Verification items for the finished model (mm, model axes). A direction names the side the tool comes from. Round coordinates to 2 decimals unless told otherwise and drop trailing zeros. Order: outer loops, then holes, each group sorted by start corner. A loop starts at its lowest first (then second) coordinate and runs counter-clockwise, first axis right, second up. Notation, with made-up numbers: (28.5, 59) -> (34.5, 59) arc R28 cw to (34.5, 77) -> close; hole circle Ø8 at (0.25, 37.5). An arc over 180 degrees is marked (long way). Put each result on its own line as item: value.
from build123d import *

# Parameters (mm, degrees)
SALIENTE_EXTRUIR1_DEPTH      = 2
SALIENTE_EXTRUIR3_DEPTH      = 2.5
SALIENTE_EXTRUIR3_DEPTH_BACK = 2
CROQUIS4_R                   = 1.5
SALIENTE_EXTRUIR4_DEPTH      = 2
CORTAR_EXTRUIR1_DEPTH        = 2


with BuildPart() as part:
    # Croquis1 → Saliente-Extruir1 (new body)
    with BuildSketch(Plane(origin=(0, 0, 0), x_dir=(1, 0, 0), z_dir=(0, 1, 0))):
        Polygon((-0.5, 44.6), (9.5, 54.6), (44.6, 54.6), (54.6, 44.6), (54.6, 9.5), (44.6, -0.5), (9.5, -0.5), (-0.5, 9.5), align=None)
    extrude(amount=SALIENTE_EXTRUIR1_DEPTH)

    # Croquis2 → Saliente-Extruir3 (add, two sides: drawn at the far end of the back side and taken through both)
    with BuildSketch(Plane(origin=(0, 2, 0), x_dir=(1, 0, 0), z_dir=(0, 1, 0)).offset(-SALIENTE_EXTRUIR3_DEPTH_BACK)):
        Polygon((7.5, 56.6), (-2.5, 46.6), (-2.5, 7.5), (7.5, -2.5), (46.6, -2.5), (56.6, 7.5), (56.6, 46.6), (46.6, 56.6), align=None)
        Polygon((44.6, -0.5), (9.5, -0.5), (-0.5, 9.5), (-0.5, 44.6), (9.5, 54.6), (44.6, 54.6), (54.6, 44.6), (54.6, 9.5), align=None, mode=Mode.SUBTRACT)
    extrude(amount=SALIENTE_EXTRUIR3_DEPTH + SALIENTE_EXTRUIR3_DEPTH_BACK)

    # Croquis4 → Saliente-Extruir4 (add)
    # profile 1 of 2: a face of its own
    with BuildSketch(Plane.XZ):
        with BuildLine():
            Line((13.025, 2.5), (21.525, 2.5))
            Line((21.525, 2.5), (21.525, 19.5))
            ThreePointArc((21.525, 19.5), (17.275, 23.75), (13.025, 19.5))
            Line((13.025, 19.5), (13.025, 2.5))
        make_face()
        with Locations(Location((17.275, 19.5, 0), (0, 0, 270))):
            Circle(CROQUIS4_R, mode=Mode.SUBTRACT)
    # profile 2 of 2: a face of its own
    with BuildSketch(Plane.XZ):
        with BuildLine():
            Line((32.575, 19.5), (32.575, 2.5))
            Line((32.575, 2.5), (41.075, 2.5))
            Line((41.075, 2.5), (41.075, 19.5))
            ThreePointArc((41.075, 19.5), (36.825, 23.75), (32.575, 19.5))
        make_face()
        with Locations(Location((36.825, 19.5, 0), (0, 0, 270))):
            Circle(CROQUIS4_R, mode=Mode.SUBTRACT)
    extrude(amount=-SALIENTE_EXTRUIR4_DEPTH)

    # Croquis6 → Cortar-Extruir1 (cut)
    with BuildSketch(Plane(origin=(0, 2, 0), x_dir=(1, 0, 0), z_dir=(0, 1, 0))):
        Polygon((4.5, 30.05), (24.05, 30.05), (24.05, 49.6), (9.5, 49.6), (4.5, 44.6), align=None)
        Polygon((30.05, 30.05), (30.05, 49.6), (44.6, 49.6), (49.6, 44.6), (49.6, 30.05), align=None)
        Polygon((30.05, 4.5), (30.05, 24.05), (49.6, 24.05), (49.6, 9.5), (44.6, 4.5), align=None)
        Polygon((9.5, 4.5), (24.05, 4.5), (24.05, 24.05), (4.5, 24.05), (4.5, 9.5), align=None)
    extrude(amount=-CORTAR_EXTRUIR1_DEPTH, mode=Mode.SUBTRACT)


solid = part.part
Item 1: Material ranges on L1, parallel to Z at x = 22, y = 0.7; L2, parallel to X at y = 0.65, z = 19.5 (3 decimals); L3, parallel to X at y = 1.85, z = 4 (3 decimals), recorded low to high. Write a range as [from, to].
Check sheet entries:
L1: z = [-56.6, -49.6], [-30.05, -24.05], [-4.5, 2.5]
L2: x = [13.025, 15.775], [18.775, 21.525], [32.575, 35.325], [38.325, 41.075]
L3: x = [13.025, 21.525], [32.575, 41.075]
Item 2: Gauge pin test, flat ends, axial feed: pin 1 Ø2.5 at (x, z) = (36.825, 19.5) entering from -Y; pin 2 Ø10 at (x, z) = (20.5, 9) entering from +Y; pin 3 Ø0.6 at (y, z) = (0.5, 13) entering from -X (3 decimals); pin 4 Ø2 at (x, y) = (35, 2.5) entering from +Z. Record the tip position at first contact, or that the pin passes through.
Check sheet entries:
pin 1: passes through
pin 2: stops at y = 2
pin 3: stops at x = 13.025
pin 4: stops at z = 23.64
Item 3: Section check D-D on x = 3.5. Record the boundary of the cut face in (y, z).
Check sheet entries:
outline: (0, -52.6) -> (4.5, -52.6) -> (4.5, -48.6) -> (2, -48.6) -> (2, -5.5) -> (4.5, -5.5) -> (4.5, -1.5) -> (0, -1.5) -> close
Item 4: Section check A-A on x = 31. Record the boundary of the cut face in (y, z), then the cut area to 3 significant figures.
Check sheet entries:
outline: (0, -56.6) -> (4.5, -56.6) -> (4.5, -54.6) -> (2, -54.6) -> (2, -49.6) -> (0, -49.6) -> close; (0, -30.05) -> (2, -30.05) -> (2, -24.05) -> (0, -24.05) -> close; (0, -4.5) -> (2, -4.5) -> (2, 0.5) -> (4.5, 0.5) -> (4.5, 2.5) -> (0, 2.5) -> close
area: 50.0 mm^2
Item 5: Section check B-B on z = -11.5. Record the boundary of the cut face in (x, y), then the cut area to 3 significant figures.
Check sheet entries:
outline: (-2.5, 0) -> (4.5, 0) -> (4.5, 2) -> (-0.5, 2) -> (-0.5, 4.5) -> (-2.5, 4.5) -> close; (24.05, 0) -> (30.05, 0) -> (30.05, 2) -> (24.05, 2) -> close; (49.6, 0) -> (56.6, 0) -> (56.6, 4.5) -> (54.6, 4.5) -> (54.6, 2) -> (49.6, 2) -> close
area: 50.0 mm^2
Item 6: Tool access check on faces 1 (the flat face through (7, 1, -47.1)), 2 (the flat face through (27, 2, -27)), 3 (the flat face through (32.575, 1, 11)), 4 (the flat face through (37, 2, 13)). Record the directions out of +Z, -Z, +X, -X, +Y, -Y that give a thin tool (end or side, any length) a straight path to the whole face; none if there is none.
Check sheet entries:
face 1: +Y, -Y
face 2: +Y
face 3: +Z, +Y, -Y
face 4: +Z, +X, -X, +Y
Item 7: Release check for a two-part mould opening along Z. For faces 5 (the flat face through (4.5, 1, -37)), 6 (the flat face through (13.025, 1, 11)), 7 (the flat face through (2.6, 2.2, -51.7)) record: +Z half, -Z half, draft (parallel to the pull), parting line (faces both ways), or undercut.
Check sheet entries:
face 5: undercut
face 6: draft
face 7: -Z half
Item 8: Section check C-C on z = 16.5. Record the boundary of the cut face in (x, y) (3 decimals), then the cut area to 3 significant figures.
Check sheet entries:
outline: (13.025, 0) -> (21.525, 0) -> (21.525, 2) -> (13.025, 2) -> close; (32.575, 0) -> (41.075, 0) -> (41.075, 2) -> (32.575, 2) -> close
area: 34.0 mm^2
